Design review of the part built by this model. Coordinates are the model's own, in mm. Face numbers are marked on the shaded views. A direction names the side the tool comes from. Give positions to 0.01 mm unless a question says otherwise; leave off trailing zeros. Write each loop counter-clockwise with the first axis right and the second up, starting at its lowest first coordinate (ties: lowest second). Pieces come first, ordered by that corner, then holes.
```python
from build123d import *

# Parameters (mm, degrees)
BOSS_EXTRUDE1_DEPTH    = 148
CONVERT_SOLID1_START   = -148
CONVERT_SOLID1_DEPTH   = 296
CONVERT_SOLID1_2_DEPTH = 296


# Read off the part's stored shape, not the designer's step: Convert-Solid1
with BuildPart() as part:
    # Sketch1 → Boss-Extrude1 (new, symmetric)
    with BuildSketch(Plane.XY):
        Polygon((0, 0), (0, 110), (17, 110), (17, 108), (2, 108), (2, 0), align=None)
    extrude(amount=BOSS_EXTRUDE1_DEPTH, both=True)

    # Convert-Solid1 outline → Convert-Solid1 (cut)
    with BuildSketch(Plane.XY.offset(CONVERT_SOLID1_START)):
        with BuildLine():
            ThreePointArc((0, 106), (1.171572875, 108.828427125), (4, 110))
            Line((4, 110), (0, 110))
            Line((0, 110), (0, 106))
        make_face()
    extrude(amount=CONVERT_SOLID1_DEPTH, mode=Mode.SUBTRACT)

    # Convert-Solid1 2 outline → Convert-Solid1 2 (add)
    with BuildSketch(Plane.XY.offset(CONVERT_SOLID1_START)):
        with BuildLine():
            ThreePointArc((2, 106), (2.585786438, 107.414213562), (4, 108))
            Line((4, 108), (2, 108))
            Line((2, 108), (2, 106))
        make_face()
    extrude(amount=CONVERT_SOLID1_2_DEPTH)


solid = part.part
```
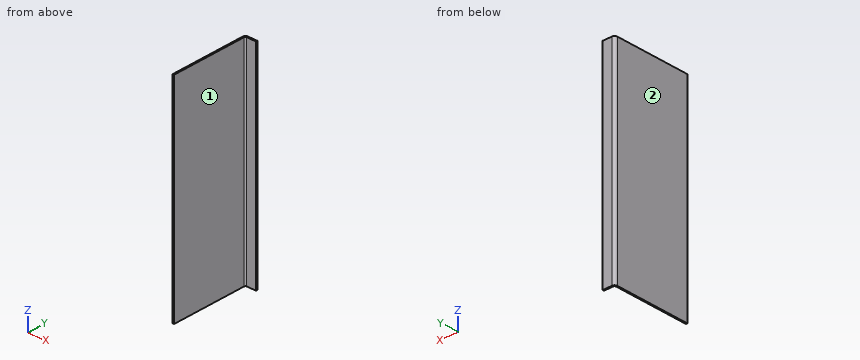
(1) Tool access review of the marked faces 1 and 2: name each direction out of +Z, -Z, +X, -X, +Y, -Y from which nothing blocks a thin tool from reaching the whole face with its end or side.
Resolved:
face 1: +Z, -Z, +X, -Y
face 2: +Z, -Z, -X, +Y, -Y
(2) Clearance check with flat-ended pins moving along their axes: P1, Ø6, axis at y = 30.5, z = -67, coming from the +X side; P2, Ø1.5, axis at x = 4, z = 6.5, coming from the -Y side; P3, Ø4, axis at x = 7.5, z = 23.5, coming from the -Y side. State where each tip first meets the part, or that it passes through.
Resolved:
P1: stops at x = 2
P2: stops at y = 107.85
P3: stops at y = 108
(3) Consider section A-A, the plane z = 26. Give the boundary of the cut face in (x, y).
Resolved:
outline: (0, 0) - (2, 0) - (2, 106) arc R2 cw to (4, 108) - (17, 108) - (17, 110) - (4, 110) arc R4 ccw to (0, 106) - close
(4) Consider section B-B, the plane x = 14.25. Give the boundary of the cut face in (y, z), then the cut area to 3 significant figures.
Resolved:
outline: (108, -148) - (110, -148) - (110, 148) - (108, 148) - close
area: 592 mm2
(5) To check wall thickness, follow L1, parallel to Y at x = 4.5, z = 130.5; L2, parallel to X at y = 15.5, z = 36; L3, parallel to Y at x = 1.5, z = -49.5. State the ranges of each line that lie inside material, in increasing order.
Resolved:
L1: y = 108 to 110
L2: x = 0 to 2
L3: y = 0 to 109.12
(6) Consider section C-C, the plane y = 37. Give the boundary of the cut face in (x, z), then the cut area to 3 significant figures.
Resolved:
outline: (0, -148) - (2, -148) - (2, 148) - (0, 148) - close
area: 592 mm2
